Source: CAD feature listing. Evaluate the final solid. Frame: model axes, mm. A direction names the side the tool comes from. Round coordinates to 2 decimals unless told otherwise and drop trailing zeros. Loops run counter-clockwise (first coordinate to the right, second up) from the corner with the lowest first, then second, coordinate; pieces in that order, holes last. Notation, with made-up numbers: M -9,-1 L 7,-1 A11 cw 7,20 Z; hole C 43,30.5 d9. An arc over 180 degrees is marked long. One line per item, written item: value.
Autodesk Inventor part; units mm, degrees
ref_plane "Work Plane2" through (-12.5, -12.5, 66.8) normal (0, 0, -1) x (0, 1, 0)
ref_plane "YZ Plane" through (0, 0, 0) normal (1, 0, 0) x (0, 1, 0)
ref_plane "XZ Plane" through (0, 0, 0) normal (0, 1, 0) x (-1, 0, 0)
ref_plane "Work Plane1" through (0, 0, 0) normal (0, 0, 1) x (1, 0, 0)
sketch "Sketch1" plane through (0, 0, 0) normal (0, 0, 1) x (1, 0, 0)
  line L0 (-30, -30) -> (30, -30)
  line L1 (30, -30) -> (30, 30)
  line L2 (30, 30) -> (-30, 30)
  line L3 (-30, 30) -> (-30, -30)
  line L4 (-30, -30) -> (30, 30) construction
  line L5 (30, -30) -> (-30, 30) construction
  circle A0 centre (-11.6, 20.0918) radius 4
  circle A1 centre (11.6, 20.0918) radius 4
  circle A2 centre (-23.2, 0) radius 4
  circle A3 centre (23.2, 0) radius 4
  circle A4 centre (11.6, -20.0918) radius 4
  circle A5 centre (-11.6, -20.0918) radius 4
  point P0 (0, 0)
  point P1 (-9.5215, -21.2918)
  dimension "d0" = 60
extrude "Extrusion1" add sketch "Sketch1" along normal blind 2
sketch "Sketch2" plane through (0, 0, 2) normal (0, 0, 1) x (1, 0, 0)
  line L0 (22.981, -22.981) -> (-22.981, -22.981) construction
  line L1 (-22.981, -22.981) -> (-22.981, 22.981) construction
  line L2 (-22.981, 22.981) -> (22.981, 22.981) construction
  line L3 (22.981, 22.981) -> (22.981, -22.981) construction
  line L4 (22.981, -22.981) -> (-22.981, 22.981) construction
  line L5 (-22.981, -22.981) -> (22.981, 22.981) construction
  circle A0 centre (0, 0) radius 32.5 construction
  circle A1 centre (-22.981, -22.981) radius 4
  circle A2 centre (22.981, -22.981) radius 4
  circle A3 centre (22.981, 22.981) radius 4
  circle A4 centre (-22.981, 22.981) radius 4
  dimension "d4" = 65
  dimension "d5" = 8
  dimension "d8" = 360
ref_plane "Work Plane2" through (-12.5, -12.5, 66.8) normal (0, 0, -1) x (0, 1, 0)
extrude "Extrusion2" add sketch "Sketch2" along normal up to surface (64.8 mm away)
sketch "Sketch3" plane through (-22.981, -22.981, 66.8) normal (0, 0, 1) x (1, 0, 0)
  line L0 (-7.019, -7.019) -> (52.981, -7.019)
  line L1 (52.981, -7.019) -> (52.981, 52.981)
  line L2 (-7.019, 52.981) -> (-7.019, -7.019)
  line L3 (52.981, 52.981) -> (-7.019, 52.981)
  circle A0 centre (5.481, 22.981) radius 2
  circle A1 centre (22.981, 40.481) radius 2
  circle A2 centre (40.481, 22.981) radius 2
  circle A3 centre (22.981, 5.481) radius 2
  arc A4 (22.0591, 26.8733) -> (26.4996, 24.8834) centre (22.981, 22.981) ccw
  circle A5 centre (22.981, 22.981) radius 4
  point P0 (22.981, 22.981)
extrude "Extrusion3" add sketch "Sketch3" against normal blind 1
sketch "Sketch4" plane through (-30, -30, 66.8) normal (0, 0, 1) x (1, 0, 0)
  line L0 (0, 60) -> (0, 0)
  line L1 (0, 0) -> (60, 0)
  line L2 (60, 0) -> (60, 60)
  line L3 (60, 60) -> (0, 60)
  circle A0 centre (30, 30) radius 4
  circle A1 centre (30, 12.5) radius 2
  circle A2 centre (47.5, 30) radius 2
  circle A3 centre (30, 47.5) radius 2
  circle A4 centre (12.5, 30) radius 2
  circle A5 centre (30, 30) radius 12.5
  point P0 (30, 30)
extrude "Extrusion4" add sketch "Sketch4" along normal blind 1 contours L3 L2 L1 L0
properties part number "mega troque motor flange for nmrv-40"
1. Section query D-D (x = -17.5). Return the cut outline in (y, z).
Report:
outline: M -30,0 L 30,0 L 30,2 L -30,2 Z; M -30,65.8 L -2,65.8 L -2,67.8 L -30,67.8 Z; M 2,65.8 L 30,65.8 L 30,67.8 L 2,67.8 Z
2. Ray query, line 1 (Y direction, x = 11.6, z = 1.05); line 2 (Y direction, x = 17.5, z = 66.65); line 3 (Z direction, x = -7.5, y = 28). Return the intervals inside material, ascending. Write a range as [from, to].
Report:
line 1: y = [-30, -24.09], [-16.09, 16.09], [24.09, 30]
line 2: y = [-30, -2], [2, 30]
line 3: z = [0, 2], [65.8, 67.8]
3. Section query C-C (y = 0). Count the separate pieces of the cut face and the enclosed holes in it, and give its area (3 significant figures).
Report:
separate pieces: 7
enclosed holes: 0
area: 159 mm2
4. Pin query (flat end, axial travel): pin 1 (6.5 mm diameter, centred on x = 11.6, y = -20.09, fed in from -Z); pin 2 (7.5 mm diameter, centred on x = 6, y = 4, fed in from +Z); pin 3 (2.5 mm diameter, centred on x = 0, y = 17.5, fed in from +Z); pin 4 (8 mm diameter, centred on x = 13, z = 39, fed in from +Y). Return the tip coordinate at first contact, or that it passes through.
Report:
pin 1: stops at z = 65.8
pin 2: stops at z = 66.8
pin 3: stops at z = 2
pin 4: passes through
5. Pull-direction query (X, two-part tool) for faces 1 (the face through (0, 0, 0)), 2 (the face through (-7.785, 18.89, 0.986)), 3 (the face through (30, 0, 67)); classes: released by +X, released by -X, zero draft, split by the parting line, or undercut.
Report:
face 1: zero draft
face 2: undercut
face 3: released by +X
6. Section query A-A (x = 0). Return the cut outline in (y, z), and give its area (3 significant figures).
Report:
outline: M -30,0 L 30,0 L 30,2 L -30,2 Z; M -30,65.8 L -19.5,65.8 L -19.5,67.8 L -30,67.8 Z; M -15.5,65.8 L -4,65.8 L -4,66.8 L -12.5,66.8 L -12.5,67.8 L -15.5,67.8 Z; M 4,65.8 L 15.5,65.8 L 15.5,67.8 L 12.5,67.8 L 12.5,66.8 L 4,66.8 Z; M 19.5,65.8 L 30,65.8 L 30,67.8 L 19.5,67.8 Z
area: 191 mm2
7. Reachability of faces 4 (the face through (-19.505, 1.532, 0.986)), 5 (the face through (15.9, 1.2, 66.8)), 6 (the face through (26.676, 24.513, 33.453)) from +Z, -Z, +X, -X, +Y, -Y: full face, straight path, thin tool, end or side. Return the list, or none.
Report:
face 4: -Z
face 5: +Z
face 6: none
8. Section query B-B (y = 13.5). Return the cut outline in (x, z), and give its area (3 significant figures).
Report:
outline: M -30,0 L 30,0 L 30,2 L -30,2 Z; M -30,65.8 L 30,65.8 L 30,67.8 L -30,67.8 Z
area: 240 mm2
